Work out the finished part from the listing and answer in its coordinate system (mm). Face numbers are marked on the shaded views. A direction names the side the tool comes from. Give positions to 0.01 mm unless a question says otherwise; leave off trailing zeros. Loops run counter-clockwise (first coordinate to the right, second up) from the corner with the lowest first, then second, coordinate; pieces in that order, holes last. Notation, with made-up numbers: (-8, -22.75) - (20, -22.75) arc R17 ccw to (20, -4.75) - close; hole circle Ø11 at (-32, -25.5). An arc over 180 degrees is marked (long way). Use CSV: the item, a comma, the result in double quotes.
from build123d import *

# Parameters (mm, degrees)
F0_R     = 2.348250802
F0_R_2   = 15
F0_W     = 3
F0_H     = 20
F0_W_2   = 42
F0_H_2   = 1
F1_DEPTH = 4
F0_W_3   = 2
F0_H_3   = 5
F2_DEPTH = 30
F4_DEPTH = 49.001
F6_DEPTH = 2
F7_DEPTH = 25
F8_R     = 3


with BuildPart() as f1:
    # F0 (on Front) → F1 (new body)
    with BuildSketch(Plane.XZ):
        Polygon((21, 14), (21, 21), (-21, 21), (-21, 14), (-21, 4), (-21, -1), (-21, -20), (21, -20), (21, -1), (21, 4), align=None)
        with Locations((-15.5, -15.5)):
            Circle(F0_R, mode=Mode.SUBTRACT)
        with Locations((15.5, -15.5)):
            Circle(F0_R, mode=Mode.SUBTRACT)
        with Locations((-15.5, 15.5)):
            Circle(F0_R, mode=Mode.SUBTRACT)
        Circle(F0_R_2, mode=Mode.SUBTRACT)
        with Locations((15.5, 15.5)):
            Circle(F0_R, mode=Mode.SUBTRACT)
        Polygon((26, -1), (21, 14), (21, 4), (23, 4), (23, -1), align=None)
        Polygon((-21, 4), (-21, 14), (-26, -1), (-23, -1), (-23, 4), align=None)
        with Locations((24.5, -11)):
            Rectangle(F0_W, F0_H)
        with Locations((-24.5, -11)):
            Rectangle(F0_W, F0_H)
        with Locations((0, -20.5)):
            Rectangle(F0_W_2, F0_H_2)
    extrude(amount=F1_DEPTH)

    # F0 (on Front) → F2 (join)
    with BuildSketch(Plane.XZ):
        with Locations((22, 1.5)):
            Rectangle(F0_W_3, F0_H_3)
        Polygon((23, -1), (21, -1), (21, -20), (21, -21), (23, -21), align=None)
        with Locations((-22, 1.5)):
            Rectangle(F0_W_3, F0_H_3)
        Polygon((-21, -20), (-21, -1), (-23, -1), (-23, -21), (-21, -21), align=None)
        with Locations((0, -20.5)):
            Rectangle(F0_W_2, F0_H_2)
    extrude(amount=F2_DEPTH)

    # F3 (on face) → F4 (cut, through all)
    with BuildSketch(Plane.YZ.offset(23)):
        Polygon((-30, -21), (-5, 4), (-30, 4), align=None)
    extrude(amount=-F4_DEPTH, mode=Mode.SUBTRACT)

    # F5 (on face) → F6 (join)
    with BuildSketch(Plane(origin=(0, 0, -21), x_dir=(1, 0, 0), z_dir=(0, 0, -1))):
        Polygon((-23, 4), (-23, 30), (-35, 30), (-26, 4), align=None)
        with BuildLine():
            ThreePointArc((-25, 28.5), (-23.9393398282, 28.0606601718), (-23.5, 27))
            ThreePointArc((-23.5, 27), (-23.9393398282, 25.9393398282), (-25, 25.5))
            Line((-25, 25.5), (-31, 25.5))
            ThreePointArc((-31, 25.5), (-32.5, 27), (-31, 28.5))
            Line((-31, 28.5), (-25, 28.5))
        make_face(mode=Mode.SUBTRACT)
        Polygon((23, 4), (26, 4), (35, 30), (23, 30), align=None)
        with BuildLine():
            ThreePointArc((25, 25.5), (23.5, 27), (25, 28.5))
            Line((25, 28.5), (31, 28.5))
            ThreePointArc((31, 28.5), (32.0606601718, 28.0606601718), (32.5, 27))
            ThreePointArc((32.5, 27), (32.0606601718, 25.9393398282), (31, 25.5))
            Line((31, 25.5), (25, 25.5))
        make_face(mode=Mode.SUBTRACT)
    extrude(amount=-F6_DEPTH)

    # F5 (on face) → F7 (cut)
    with BuildSketch(Plane(origin=(0, 0, -21), x_dir=(1, 0, 0), z_dir=(0, 0, -1))):
        with BuildLine():
            ThreePointArc((-7, 7), (-8.5, 8.5), (-7, 10))
            Line((-7, 10), (-13, 10))
            ThreePointArc((-13, 10), (-11.9393398282, 9.5606601718), (-11.5, 8.5))
            ThreePointArc((-11.5, 8.5), (-11.9393398282, 7.4393398282), (-13, 7))
            Line((-13, 7), (-7, 7))
        make_face()
        with BuildLine():
            ThreePointArc((-11.5, 8.5), (-11.9393398282, 9.5606601718), (-13, 10))
            ThreePointArc((-13, 10), (-14.5, 8.5), (-13, 7))
            ThreePointArc((-13, 7), (-11.9393398282, 7.4393398282), (-11.5, 8.5))
        make_face()
        with BuildLine():
            ThreePointArc((-7, 7), (-5.9393398282, 7.4393398282), (-5.5, 8.5))
            ThreePointArc((-5.5, 8.5), (-5.9393398282, 9.5606601718), (-7, 10))
            ThreePointArc((-7, 10), (-8.5, 8.5), (-7, 7))
        make_face()
        with BuildLine():
            Line((13, 10), (7, 10))
            ThreePointArc((7, 10), (8.0606601718, 9.5606601718), (8.5, 8.5))
            ThreePointArc((8.5, 8.5), (8.0606601718, 7.4393398282), (7, 7))
            Line((7, 7), (13, 7))
            ThreePointArc((13, 7), (11.5, 8.5), (13, 10))
        make_face()
        with BuildLine():
            ThreePointArc((14.5, 8.5), (14.0606601718, 9.5606601718), (13, 10))
            ThreePointArc((13, 10), (11.5, 8.5), (13, 7))
            ThreePointArc((13, 7), (14.0606601718, 7.4393398282), (14.5, 8.5))
        make_face()
        with BuildLine():
            ThreePointArc((8.5, 8.5), (8.0606601718, 9.5606601718), (7, 10))
            ThreePointArc((7, 10), (5.5, 8.5), (7, 7))
            ThreePointArc((7, 7), (8.0606601718, 7.4393398282), (8.5, 8.5))
        make_face()
    extrude(amount=-F7_DEPTH, mode=Mode.SUBTRACT)

    # F8
    f8_edges = [f1.edges().sort_by_distance(p)[0] for p in [
        (21, -2, 21),
        (-21, -2, 21),
    ]]
    fillet(f8_edges, radius=F8_R)


solid = f1.part
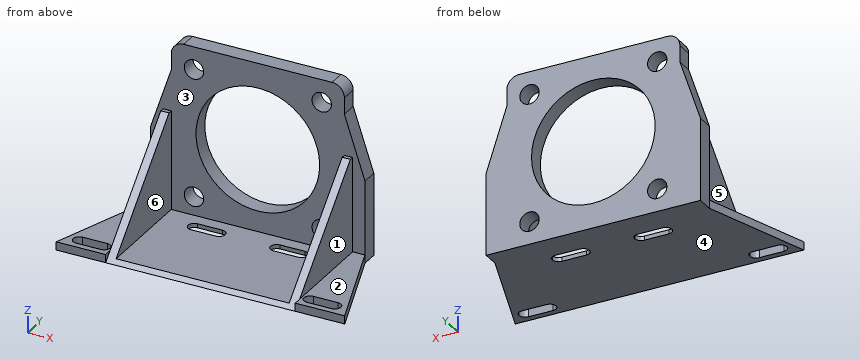
Item 1: A cutting plane is placed at C-C on y = -2.5. Determine the outline of the cut face in (x, z), and give its area (3 significant figures).
Determined:
outline,"(-26, -21) - (26, -21) - (26, -1) - (21, 14) - (21, 18) arc R3 ccw to (18, 21) - (-18, 21) arc R3 ccw to (-21, 18) - (-21, 14) - (-26, -1) - close; hole circle Ø4.7 at (-15.5, -15.5); hole circle Ø4.7 at (-15.5, 15.5); hole circle Ø30 at (0, 0); hole circle Ø4.7 at (15.5, -15.5); hole circle Ø4.7 at (15.5, 15.5)"
area,"1,260 mm²"
Item 2: Given P1, Ø12.5, axis at x = -10, z = -5, coming from the -Y side; P2, Ø0.5, axis at x = -10.5, z = -20.5, coming from the -Y side; P3, Ø1.5, axis at x = -10, z = -15, coming from the +Y side; P4, Ø3, axis at x = -15.5, z = -15.5, coming from the -Y side, each flat-ended and moving along its own axis, determine where each tip first touches the part or whether it passes through.
Determined:
P1,"stops at y = -4"
P2,"stops at y = -29.75"
P3,"stops at y = 0"
P4,"passes through"
Item 3: A cutting plane is placed at D-D on x = 10. Determine the outline of the cut face in (y, z).
Determined:
outline,"(-30, -21) - (-10, -21) - (-10, -20) - (-29, -20) - close; (-7, -21) - (0, -21) - (0, -11.18) - (-4, -11.18) - (-4, -20) - (-7, -20) - close; (-4, 11.18) - (0, 11.18) - (0, 21) - (-4, 21) - close"
Item 4: A cutting plane is placed at B-B on z = -3. Determine the outline of the cut face in (x, y).
Determined:
outline,"(-26, -4) - (-23, -4) - (-23, -12) - (-21, -12) - (-21, -4) - (-14.7, -4) - (-14.7, 0) - (-26, 0) - close; (14.7, -4) - (21, -4) - (21, -12) - (23, -12) - (23, -4) - (26, -4) - (26, 0) - (14.7, 0) - close"
Item 5: For the marked faces 4, 5 and 6, determine the directions among +Z, -Z, +X, -X, +Y, -Y from which every point of the face is accessible in a straight line to the end or side of a thin tool.
Determined:
face 4,"-Z, +X, -X, +Y, -Y"
face 5,"+Z, -X, -Y"
face 6,"+Z, -Y"
Item 6: A cutting plane is placed at A-A on x = 0. Determine the outline of the cut face in (y, z).
Determined:
outline,"(-30, -21) - (0, -21) - (0, -15) - (-4, -15) - (-4, -20) - (-29, -20) - close; (-4, 15) - (0, 15) - (0, 21) - (-4, 21) - close"
Item 7: The mould has two halves that part along X. Classify the marked faces 1, 2 and 3: pulls with the +X half, pulls with the -X half, needs draft (parallel to the pull), parting line crosses it, or undercut.
Determined:
face 1,"pulls with the +X half"
face 2,"needs draft"
face 3,"undercut"
Item 8: Find the intervals of material crossed by line 1 (Z direction, x = -15.5, y = -2); line 2 (X direction, y = -6.5, z = -16.5); line 3 (Z direction, x = 0, y = -1.4), in increasing order.
Determined:
line 1,"z = -21 to -17.85, -13.15 to 13.15, 17.85 to 21"
line 2,"x = -23 to -21, 21 to 23"
line 3,"z = -21 to -15, 15 to 21"
